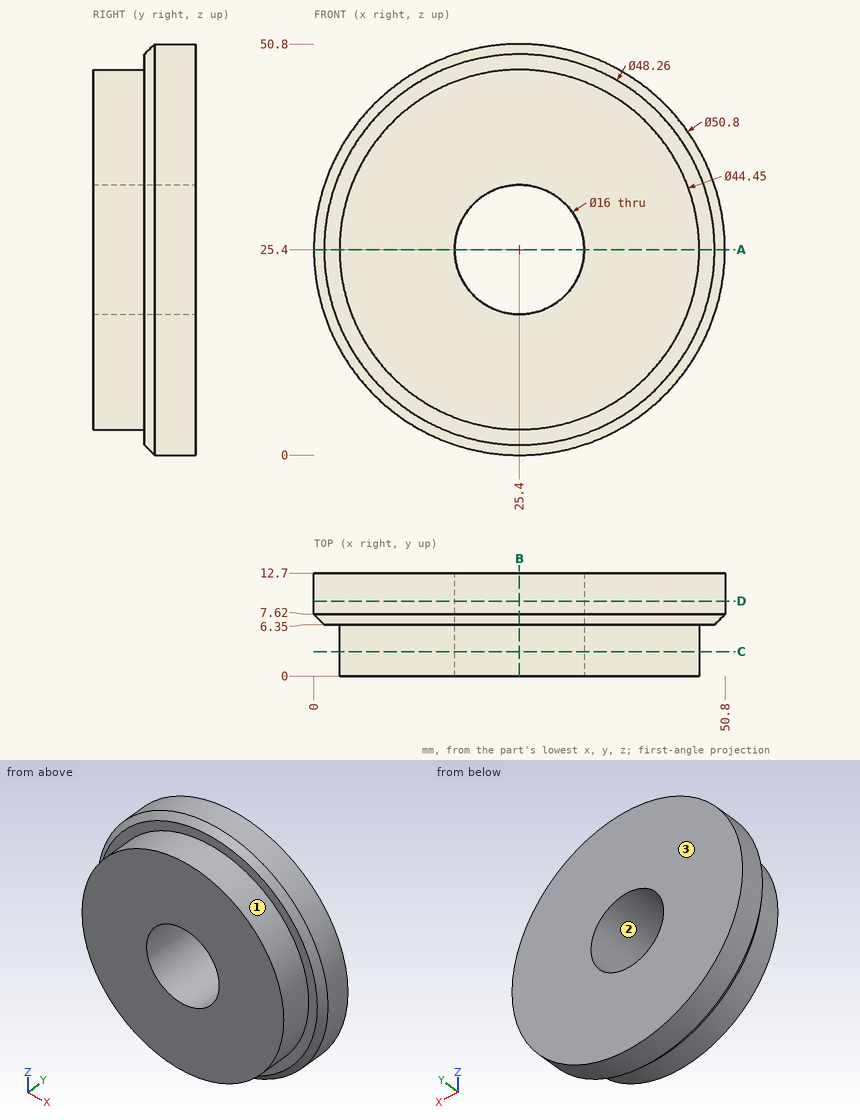
Drawing for the job (mm, zero at the part's lowest x, y, z). Round coordinates to 2 decimals unless told otherwise and drop trailing zeros. Loops run counter-clockwise (first coordinate to the right, second up) from the corner with the lowest first, then second, coordinate; pieces in that order, holes last. Notation, with made-up numbers: (15, 10) -> (73, 10) arc R32 ccw to (73, 37) -> close; hole circle Ø7 at (16.5, 5). An arc over 180 degrees is marked (long way). Answer in a Markdown table with one row per item.
Item 1: Saw through at B-B (x = 25.4). Write the cut outline in (y, z) (3 decimals), and give its area (3 significant figures).
Answers below:
| item | result |
|---|---|
| outline | (0, 3.175) -> (6.35, 3.175) -> (6.35, 1.27) -> (7.62, 0) -> (12.7, 0) -> (12.7, 17.4) -> (0, 17.4) -> close; (0, 33.4) -> (12.7, 33.4) -> (12.7, 50.8) -> (7.62, 50.8) -> (6.35, 49.53) -> (6.35, 47.625) -> (0, 47.625) -> close |
| area | 400 mm² |
Item 2: Saw through at A-A (z = 25.4). Write the cut outline in (x, y) (3 decimals).
Answers below:
| item | result |
|---|---|
| outline | (0, 7.62) -> (1.27, 6.35) -> (3.175, 6.35) -> (3.175, 0) -> (17.4, 0) -> (17.4, 12.7) -> (0, 12.7) -> close; (33.4, 0) -> (47.625, 0) -> (47.625, 6.35) -> (49.53, 6.35) -> (50.8, 7.62) -> (50.8, 12.7) -> (33.4, 12.7) -> close |
Item 3: Saw through at C-C (y = 3). Write the cut outline in (x, z) (3 decimals).
Answers below:
| item | result |
|---|---|
| outline | circle Ø44.45 at (25.4, 25.4); hole circle Ø16 at (25.4, 25.4) |
Item 4: Drill centre lines: L1, parallel to Z at x = 25.4, y = 10; L2, parallel to Z at x = 25.4, y = 5.25 (3 decimals); L3, parallel to Y at x = 47, z = 31. Where is each one in solid material? Low to high. Write a range as [from, to].
Answers below:
| item | result |
|---|---|
| L1 | z = [0, 17.4], [33.4, 50.8] |
| L2 | z = [3.175, 17.4], [33.4, 47.625] |
| L3 | y = [6.35, 12.7] |
Item 5: Pin check, flat tips, straight feed: pin 1 (6 mm diameter, centred on y = 2, z = 35, fed in from +X); pin 2 (1.5 mm diameter, centred on x = 43, z = 44, fed in from +Y); pin 3 (2 mm diameter, centred on x = 44.5, y = 2, fed in from -Z); pin 4 (1.5 mm diameter, centred on y = 5, z = 15.5, fed in from +X). Stop position of each tip, or through.
Answers below:
| item | result |
|---|---|
| pin 1 | stops at x = 46.62 |
| pin 2 | stops at y = 12.7 |
| pin 3 | stops at z = 12.5 |
| pin 4 | stops at x = 45.65 |
Item 6: Saw through at D-D (y = 9.25). Write the cut outline in (x, z), and give its area (3 significant figures).
Answers below:
| item | result |
|---|---|
| outline | circle Ø50.8 at (25.4, 25.4); hole circle Ø16 at (25.4, 25.4) |
| area | 1,830 mm² |
Item 7: Mould opens along X. For the marked faces 1, 2 and 3 say: +X half, -X half, draft (parallel to the pull), parting line (faces both ways), or undercut.
Answers below:
| item | result |
|---|---|
| face 1 | parting line |
| face 2 | undercut |
| face 3 | draft |
